For this review, take the finished solid that the model builds, in its own axes (mm). A direction names the side the tool comes from. Round coordinates to 2 decimals unless told otherwise and drop trailing zeros. Write each loop counter-clockwise with the first axis right and the second up, starting at its lowest first coordinate (ties: lowest second). Pieces come first, ordered by that corner, then holes. Notation, with made-up numbers: (56, 5.5) -> (92, 5.5) arc R20 cw to (92, 27.5) -> close; hole circle Ø1 at (47.5, -23.5). An arc over 180 degrees is marked (long way). Write each question's results on one line, items separated by ' | '. Start each with the question number.
Item 1: Add section B-B (y = 48.6). State the section outline as (x, z) points, plus the area to 3 significant figures.
Item 2: Add section A-A (z = 0). State the section outline as (x, y) points.
Item 3: Tool access review of faces 5 (the flat face through (-32, 30, 11.3)), 6 (the flat face through (-21.1, 11.7, -12.5)), 7 (the flat face through (-28.2, 48, 0)), 8 (the cylindrical face through (-29.2, 61, 6.5)): name each direction out of +Z, -Z, +X, -X, +Y, -Y from which nothing blocks a thin tool from reaching the whole face with its end or side.
Item 4: Add section D-D (y = 56.5). State the section outline as (x, z) points, plus the area to 3 significant figures.
Item 5: Add section C-C (x = -8). State the section outline as (y, z) points.
Item 6: The part is to be moulded in two halves that separate along Y. For faces 1 (the flat face through (-21.1, 11.6, 12.5)), 2 (the flat face through (-32.2, 19.5, -11.9)), 3 (the flat face through (0, 0, 0)), 4 (the flat face through (13, 9.6, -3)), say which applies: +Y half, -Y half, draft (parallel to the pull), parting line (faces both ways), or undercut.
Item 7: To check wall thickness, follow line 1 along X through (y, z) = (47, -1); line 2 along Y through (x, z) = (2, -16); line 3 along Y through (x, z) = (-2, 12). State the ranges of each line that lie inside material, in increasing order.
Item 8: Clearance check with flat-ended pins moving along their axes: pin 1 (2 mm diameter, centred on x = -19.5, y = 11.5, fed in from -Z); pin 2 (8 mm diameter, centred on y = 55, z = -9.5, fed in from +X); pin 3 (2 mm diameter, centred on y = 30.5, z = 7.5, fed in from +X); pin 4 (11 mm diameter, centred on x = -18.5, z = -5.5, fed in from -Y). State where each tip first meets the part, or that it passes through.
from build123d import *

# Parameters (mm, degrees)
SKETCH1_R           = 17.4
BOSS_EXTRUDE1_DEPTH = 9.6
BOSS_EXTRUDE2_DEPTH = 2.4
BOSS_EXTRUDE3_DEPTH = 4
SKETCH6_R           = 14
BOSS_EXTRUDE4_DEPTH = 4
BOSS_EXTRUDE5_START = 2
SKETCH7_R           = 14
BOSS_EXTRUDE5_DEPTH = 2


with BuildPart() as part:
    # Sketch1 → Boss-Extrude1 (new body)
    with BuildSketch(Plane(origin=(0, 0, 0), x_dir=(1, 0, 0), z_dir=(0, 1, 0))):
        with Locations(Location((0, 0, 0), (0, 0, 270))):
            Circle(SKETCH1_R)
    extrude(amount=BOSS_EXTRUDE1_DEPTH)

    # Sketch2 → Boss-Extrude2 (add)
    with BuildSketch(Plane(origin=(0, 9.6, 0), x_dir=(1, 0, 0), z_dir=(0, 1, 0))):
        with BuildLine():
            Line((0, -12.5), (-34.2, -12.5))
            Line((-34.2, -12.5), (-34.2, 12.5))
            Line((-34.2, 12.5), (0, 12.5))
            ThreePointArc((0, 12.5), (12.5, 0), (0, -12.5))
        make_face()
    extrude(amount=BOSS_EXTRUDE2_DEPTH)

    # Sketch5 → Boss-Extrude3 (add)
    with BuildSketch(Plane.ZY.offset(34.2)):
        with BuildLine():
            Line((11.3, 22), (11.3, 38.137208785))
            ThreePointArc((11.3, 38.137208785), (0, 64), (-11.3, 38.137208785))
            Line((-11.3, 38.137208785), (-11.3, 22))
            Line((-11.3, 22), (-12.5, 17))
            Line((-12.5, 17), (-12.5, 12))
            Line((-12.5, 12), (12.5, 12))
            Line((12.5, 12), (12.5, 17))
            Line((12.5, 17), (11.3, 22))
        make_face()
    extrude(amount=-BOSS_EXTRUDE3_DEPTH)

    # Sketch6 → Boss-Extrude4 (add)
    with BuildSketch(Plane.ZY.offset(34.2)):
        with Locations((0, 48.6)):
            Circle(SKETCH6_R)
    extrude(amount=BOSS_EXTRUDE4_DEPTH)

    # Sketch7 → Boss-Extrude5 (add)
    with BuildSketch(Plane(origin=(-30.2, 0, 0), x_dir=(0, 0, -1), z_dir=(1, 0, 0)).offset(BOSS_EXTRUDE5_START)):
        with Locations(Location((0, 48.6, 0), (0, 0, 180))):
            Circle(SKETCH7_R)
    extrude(amount=-BOSS_EXTRUDE5_DEPTH)


solid = part.part
Responses:
1) outline: (-38.2, -14) -> (-34.2, -14) -> (-34.2, -15.4) -> (-30.2, -15.4) -> (-30.2, -14) -> (-28.2, -14) -> (-28.2, 14) -> (-30.2, 14) -> (-30.2, 15.4) -> (-34.2, 15.4) -> (-34.2, 14) -> (-38.2, 14) -> close | area: 291 mm^2
2) outline: (-38.2, 34.6) -> (-34.2, 34.6) -> (-34.2, 9.6) -> (-17.4, 9.6) -> (-17.4, 0) -> (17.4, 0) -> (17.4, 9.6) -> (12.5, 9.6) -> (12.5, 12) -> (-30.2, 12) -> (-30.2, 34.6) -> (-28.2, 34.6) -> (-28.2, 62.6) -> (-30.2, 62.6) -> (-30.2, 64) -> (-34.2, 64) -> (-34.2, 62.6) -> (-38.2, 62.6) -> close
3) face 5: +Z, +X, -X | face 6: -Z, +X, -X | face 7: +Z, -Z, +X, +Y | face 8: +X
4) outline: (-38.2, -11.56) -> (-34.2, -11.56) -> (-34.2, -13.22) -> (-30.2, -13.22) -> (-30.2, -11.56) -> (-28.2, -11.56) -> (-28.2, 11.56) -> (-30.2, 11.56) -> (-30.2, 13.22) -> (-34.2, 13.22) -> (-34.2, 11.56) -> (-38.2, 11.56) -> close | area: 244 mm^2
5) outline: (0, -15.45) -> (9.6, -15.45) -> (9.6, -12.5) -> (12, -12.5) -> (12, 12.5) -> (9.6, 12.5) -> (9.6, 15.45) -> (0, 15.45) -> close
6) face 1: draft | face 2: undercut | face 3: -Y half | face 4: +Y half
7) line 1: x = -38.2 to -28.2 | line 2: y = 0 to 9.6 | line 3: y = 0 to 12
8) pin 1: stops at z = -12.5 | pin 2: stops at x = -28.2 | pin 3: stops at x = -30.2 | pin 4: stops at y = 0
